Could you check a few things on this model? Use its own coordinates, in mm. A direction names the side the tool comes from. Give positions to 0.01 mm unless a question says otherwise; leave off trailing zeros. Write each loop counter-clockwise with the first axis right and the second up, starting at its lowest first coordinate (ties: lowest second). Pieces come first, ordered by that corner, then holes. Notation, with made-up numbers: (26, 76.25) - (71, 76.25) arc R12 ccw to (71, 86.25) - close; hole circle Ø4 at (-38, -28). An arc over 180 degrees is marked (long way). Use one line per item in the form item = value.
```python
from build123d import *

# Parameters (mm, degrees)
BOSS_EXTRUDE1_DEPTH = 1.8
SKETCH2_R           = 25
CUT_EXTRUDE1_DEPTH  = 1.8
SKETCH2_3_R         = 4.5
BOSS_EXTRUDE2_DEPTH = 4
SKETCH2_4_R         = 4.5
SKETCH2_4_R_2       = 3
CUT_EXTRUDE2_DEPTH  = 2
CIRPATTERN1_COUNT   = 12
SKETCH5_W           = 3
SKETCH5_H           = 8
CUT_EXTRUDE3_DEPTH  = 1.8


with BuildPart() as part:
    # Sketch1 → Boss-Extrude1 (new body)
    with BuildSketch(Plane(origin=(0, 0, 0), x_dir=(1, 0, 0), z_dir=(0, 1, 0))):
        with BuildLine():
            Line((-50, 0), (-50, -50))
            Line((-50, -50), (50, -50))
            Line((50, -50), (50, 0))
            ThreePointArc((50, 0), (0, 50), (-50, 0))
        make_face()
    extrude(amount=BOSS_EXTRUDE1_DEPTH)

    # Sketch2 → Cut-Extrude1 (cut)
    with BuildSketch(Plane(origin=(0, 1.8, 0), x_dir=(1, 0, 0), z_dir=(0, 1, 0))):
        with Locations(Location((0, 0, 0), (0, 0, 270))):
            Circle(SKETCH2_R)
    extrude(amount=-CUT_EXTRUDE1_DEPTH, mode=Mode.SUBTRACT)

    # Sketch2<3> → Boss-Extrude2 (add)
    with BuildSketch(Plane(origin=(0, 1.8, 0), x_dir=(1, 0, 0), z_dir=(0, 1, 0))):
        with Locations(Location((0, -40, 0), (0, 0, 270))):
            Circle(SKETCH2_3_R)
    boss_extrude2 = extrude(amount=BOSS_EXTRUDE2_DEPTH)

    # Sketch2<4> → Cut-Extrude2 (cut)
    with BuildSketch(Plane(origin=(0, 1.8, 0), x_dir=(1, 0, 0), z_dir=(0, 1, 0))):
        with Locations(Location((0, -40, 0), (0, 0, 270))):
            Circle(SKETCH2_4_R)
        with Locations(Location((0, -40, 0), (0, 0, 270))):
            Circle(SKETCH2_4_R_2, mode=Mode.SUBTRACT)
    cut_extrude2 = extrude(amount=CUT_EXTRUDE2_DEPTH, mode=Mode.SUBTRACT)

    # CirPattern1: Boss-Extrude2, Cut-Extrude2 ×12 about axis, 6 skipped
    cirpattern1_axis = Axis((0, -70.710678119, 0), (0, 1, 0))
    add([boss_extrude2.rotate(cirpattern1_axis, i * 360 / CIRPATTERN1_COUNT) for i in range(1, CIRPATTERN1_COUNT) if i not in (1, 3, 5, 7, 9, 11)])
    add([cut_extrude2.rotate(cirpattern1_axis, i * 360 / CIRPATTERN1_COUNT) for i in range(1, CIRPATTERN1_COUNT) if i not in (1, 3, 5, 7, 9, 11)], mode=Mode.SUBTRACT)

    # Sketch5 → Cut-Extrude3 (cut)
    with BuildSketch(Plane(origin=(0, 1.8, 0), x_dir=(1, 0, 0), z_dir=(0, 1, 0))):
        with Locations((-45.5, 0)):
            Rectangle(SKETCH5_W, SKETCH5_H)
        with Locations((45.5, 0)):
            Rectangle(SKETCH5_W, SKETCH5_H)
    extrude(amount=-CUT_EXTRUDE3_DEPTH, mode=Mode.SUBTRACT)


solid = part.part
```
1. Imagine slicing it at D-D, the plane x = -35.5. List the corners of the cut face in (y, z) for me, and give its area (3 significant figures).
Response values:
outline = (0, -35.21) - (1.8, -35.21) - (1.8, -22.87) - (3.8, -22.87) - (3.8, -24.42) - (5.8, -24.42) - (5.8, -15.58) - (3.8, -15.58) - (3.8, -17.13) - (1.8, -17.13) - (1.8, 17.13) - (3.8, 17.13) - (3.8, 15.58) - (5.8, 15.58) - (5.8, 24.42) - (3.8, 24.42) - (3.8, 22.87) - (1.8, 22.87) - (1.8, 50) - (0, 50) - close
area = 212 mm²
2. Which directions (+Z, -Z, +X, -X, +Y, -Y) give clear straight access to the entire face, cutting with the end or side of a thin tool? Please do faces 1 (the face through (-35, 5.8, 20)), 2 (the face through (30.847, 4.786, 17.581)), 3 (the face through (32.6, 2.8, 22.2)).
Response values:
face_1 = +Z, -Z, +X, -X, +Y
face_2 = +Y
face_3 = none
3. Imagine slicing it at B-B, the plane x = 0. List the corners of the cut face in (y, z) for me.
Response values:
outline = (0, -50) - (1.8, -50) - (1.8, -43) - (3.8, -43) - (3.8, -44.5) - (5.8, -44.5) - (5.8, -35.5) - (3.8, -35.5) - (3.8, -37) - (1.8, -37) - (1.8, -25) - (0, -25) - close; (0, 25) - (1.8, 25) - (1.8, 37) - (3.8, 37) - (3.8, 35.5) - (5.8, 35.5) - (5.8, 44.5) - (3.8, 44.5) - (3.8, 43) - (1.8, 43) - (1.8, 50) - (0, 50) - close
4. If we mould it in two halves opening along X, with no side actions, what happens to faces 4 (the face through (0, 5.8, -40)), 5 (the face through (1.099, 0.887, -49.988)), 6 (the face through (7.509, 0.913, 23.846))? For each: pulls with the +X half, pulls with the -X half, needs draft (parallel to the pull), parting line crosses it, or undercut.
Response values:
face_4 = needs draft
face_5 = parting line crosses it
face_6 = undercut
5. Imagine slicing it at A-A, the plane z = 20. List the corners of the cut face in (x, y) for me, and give its area (3 significant figures).
Response values:
outline = (-50, 0) - (-15, 0) - (-15, 1.8) - (-31.64, 1.8) - (-31.64, 3.8) - (-30.14, 3.8) - (-30.14, 5.8) - (-39.14, 5.8) - (-39.14, 3.8) - (-37.64, 3.8) - (-37.64, 1.8) - (-50, 1.8) - close; (15, 0) - (50, 0) - (50, 1.8) - (37.64, 1.8) - (37.64, 3.8) - (39.14, 3.8) - (39.14, 5.8) - (30.14, 5.8) - (30.14, 3.8) - (31.64, 3.8) - (31.64, 1.8) - (15, 1.8) - close
area = 186 mm²
6. Imagine slicing it at C-C, the plane z = 40. List the corners of the cut face in (x, y) for me.
Response values:
outline = (-50, 0) - (50, 0) - (50, 1.8) - (3, 1.8) - (3, 3.8) - (4.5, 3.8) - (4.5, 5.8) - (-4.5, 5.8) - (-4.5, 3.8) - (-3, 3.8) - (-3, 1.8) - (-50, 1.8) - close
7. For pin 1 (0.5 mm diameter, centred on x = -45.5, y = 1, fed in from -Z); pin 2 (1.5 mm diameter, centred on y = 4.5, z = -4.5, fed in from +X); pin 3 (0.5 mm diameter, centred on x = 46, y = 0.5, fed in from -Z); pin 4 (1 mm diameter, centred on x = -33, z = 6, fed in from +Y), each with a flat end and sliding along its axis, tell me the tip position at first contact or that it passes through.
Response values:
pin_1 = -21.27
pin_2 = through
pin_3 = -20.17
pin_4 = 1.8
8. If I drill on line 1 (X direction, y = 1.2, z = 0); line 2 (Y direction, x = 2, z = -26.5); line 3 (X direction, y = 5.05, z = 16), over which ranges is the centre line in solid material (lowest first)? Write a range as from..to.
Response values:
line_1 = -50..-47, -44..-25, 25..44, 47..50
line_2 = 0..1.8
line_3 = -36.7..-32.58, 32.58..36.7
